Work out the finished part from the listing and answer in its coordinate system (mm). A direction names the side the tool comes from. Give positions to 0.01 mm unless a question says otherwise; leave off trailing zeros. Loops run counter-clockwise (first coordinate to the right, second up) from the corner with the lowest first, then second, coordinate; pieces in that order, holes last. Notation, with made-up numbers: M 78,-34 L 100,-34 A26 ccw 100,-10 Z; hole C -29,-37 d5. An arc over 180 degrees is marked long. Answer in a Markdown table with one row per item. Add a question column.
from build123d import *

# Parameters (mm, degrees)
SKETCH2_W           = 130
SKETCH2_H           = 40
BOSS_EXTRUDE1_DEPTH = 75
SKETCH6_W           = 29.16
SKETCH6_H           = 49.32
BOSS_EXTRUDE2_DEPTH = 16.07
SKETCH7_W           = 15.96
SKETCH7_H           = 42.65
CUT_EXTRUDE1_DEPTH  = 8.48
SKETCH8_W           = 7
SKETCH8_H           = 42.65
CUT_EXTRUDE2_DEPTH  = 1.145
SKETCH9_W           = 7
SKETCH9_H           = 42.65
CUT_EXTRUDE3_DEPTH  = 1.145
SKETCH11_W          = 35.86
SKETCH11_H          = 21.1
CUT_EXTRUDE4_DEPTH  = 8.2
SKETCH13_W          = 3.9
SKETCH13_H          = 21.1
CUT_EXTRUDE5_DEPTH  = 1.145
SKETCH14_W          = 3.9
SKETCH14_H          = 21.1
CUT_EXTRUDE6_DEPTH  = 1.145
SKETCH15_W          = 35.86
SKETCH15_H          = 21.1
CUT_EXTRUDE7_DEPTH  = 8.2
SKETCH16_W          = 3.9
SKETCH16_H          = 21.1
CUT_EXTRUDE8_DEPTH  = 1.145
SKETCH17_W          = 3.9
SKETCH17_H          = 21.1
CUT_EXTRUDE9_DEPTH  = 1.145
SKETCH20_W          = 29.16
SKETCH20_H          = 16.07
BOSS_EXTRUDE3_DEPTH = 25.68
SKETCH21_W          = 40
SKETCH21_H          = 25
CUT_EXTRUDE10_DEPTH = 40
SKETCH22_W          = 50
SKETCH22_H          = 25
CUT_EXTRUDE11_DEPTH = 40
BOSS_EXTRUDE4_DEPTH = 8
BOSS_EXTRUDE5_DEPTH = 8


with BuildPart() as part:
    # Sketch2 → Boss-Extrude1 (new body)
    with BuildSketch(Plane(origin=(0, 0, 0), x_dir=(1, 0, 0), z_dir=(0, 1, 0))):
        Rectangle(SKETCH2_W, SKETCH2_H)
    extrude(amount=BOSS_EXTRUDE1_DEPTH)

    # Sketch6 → Boss-Extrude2 (add)
    with BuildSketch(Plane.XY.offset(20)):
        with Locations((0, 50.34)):
            Rectangle(SKETCH6_W, SKETCH6_H)
    extrude(amount=BOSS_EXTRUDE2_DEPTH)

    # Sketch7 → Cut-Extrude1 (cut)
    with BuildSketch(Plane.XY.offset(36.07)):
        with Locations((0, 53.675)):
            Rectangle(SKETCH7_W, SKETCH7_H)
    extrude(amount=-CUT_EXTRUDE1_DEPTH, mode=Mode.SUBTRACT)

    # Sketch8 → Cut-Extrude2 (cut)
    with BuildSketch(Plane(origin=(-7.98, 0, 0), x_dir=(0, 0, -1), z_dir=(1, 0, 0))):
        with Locations((-31.09, 53.675)):
            Rectangle(SKETCH8_W, SKETCH8_H)
    extrude(amount=-CUT_EXTRUDE2_DEPTH, mode=Mode.SUBTRACT)

    # Sketch9 → Cut-Extrude3 (cut)
    with BuildSketch(Plane.ZY.offset(-7.98)):
        with Locations((31.09, 53.675)):
            Rectangle(SKETCH9_W, SKETCH9_H)
    extrude(amount=-CUT_EXTRUDE3_DEPTH, mode=Mode.SUBTRACT)

    # Sketch11 → Cut-Extrude4 (cut)
    with BuildSketch(Plane.XY.offset(20)):
        with Locations((42.64, 64.45)):
            Rectangle(SKETCH11_W, SKETCH11_H)
    extrude(amount=-CUT_EXTRUDE4_DEPTH, mode=Mode.SUBTRACT)

    # Sketch13 → Cut-Extrude5 (cut)
    with BuildSketch(Plane(origin=(24.71, 0, 0), x_dir=(0, 0, -1), z_dir=(1, 0, 0))):
        with Locations((-13.75, 64.45)):
            Rectangle(SKETCH13_W, SKETCH13_H)
    extrude(amount=-CUT_EXTRUDE5_DEPTH, mode=Mode.SUBTRACT)

    # Sketch14 → Cut-Extrude6 (cut)
    with BuildSketch(Plane.ZY.offset(-60.57)):
        with Locations((13.75, 64.45)):
            Rectangle(SKETCH14_W, SKETCH14_H)
    extrude(amount=-CUT_EXTRUDE6_DEPTH, mode=Mode.SUBTRACT)

    # Sketch15 → Cut-Extrude7 (cut)
    with BuildSketch(Plane.XY.offset(20)):
        with Locations((-42.64, 64.45)):
            Rectangle(SKETCH15_W, SKETCH15_H)
    extrude(amount=-CUT_EXTRUDE7_DEPTH, mode=Mode.SUBTRACT)

    # Sketch16 → Cut-Extrude8 (cut)
    with BuildSketch(Plane(origin=(-60.57, 0, 0), x_dir=(0, 0, -1), z_dir=(1, 0, 0))):
        with Locations((-13.75, 64.45)):
            Rectangle(SKETCH16_W, SKETCH16_H)
    extrude(amount=-CUT_EXTRUDE8_DEPTH, mode=Mode.SUBTRACT)

    # Sketch17 → Cut-Extrude9 (cut)
    with BuildSketch(Plane.ZY.offset(24.71)):
        with Locations((13.75, 64.45)):
            Rectangle(SKETCH17_W, SKETCH17_H)
    extrude(amount=-CUT_EXTRUDE9_DEPTH, mode=Mode.SUBTRACT)

    # Sketch20 → Boss-Extrude3 (add)
    with BuildSketch(Plane(origin=(0, 25.68, 0), x_dir=(-1, 0, 0), z_dir=(0, -1, 0))):
        with Locations((0, -28.035)):
            Rectangle(SKETCH20_W, SKETCH20_H)
    extrude(amount=BOSS_EXTRUDE3_DEPTH)

    # Sketch21 → Cut-Extrude10 (cut)
    with BuildSketch(Plane(origin=(0, 75, 0), x_dir=(1, 0, 0), z_dir=(0, 1, 0))):
        with Locations((45, 7.5)):
            Rectangle(SKETCH21_W, SKETCH21_H)
        with Locations((-45, 7.5)):
            Rectangle(SKETCH21_W, SKETCH21_H)
    extrude(amount=-CUT_EXTRUDE10_DEPTH, mode=Mode.SUBTRACT)

    # Sketch22 → Cut-Extrude11 (cut)
    with BuildSketch(Plane(origin=(0, 75, 0), x_dir=(1, 0, 0), z_dir=(0, 1, 0))):
        with Locations((0, 7.5)):
            Rectangle(SKETCH22_W, SKETCH22_H)
    extrude(amount=-CUT_EXTRUDE11_DEPTH, mode=Mode.SUBTRACT)

    # Sketch23 → Boss-Extrude4 (add)
    with BuildSketch(Plane(origin=(0, 53.9, 0), x_dir=(1, 0, 0), z_dir=(0, 1, 0))):
        Polygon((-60.57, -20), (-60.57, -15.7), (-61.715, -15.7), (-61.715, -11.8), (-23.565, -11.8), (-23.565, -15.7), (-24.71, -15.7), (-24.71, -20), align=None)
    extrude(amount=BOSS_EXTRUDE4_DEPTH)

    # Sketch24 → Boss-Extrude5 (add)
    with BuildSketch(Plane(origin=(0, 53.9, 0), x_dir=(1, 0, 0), z_dir=(0, 1, 0))):
        Polygon((24.71, -20), (24.71, -15.7), (23.565, -15.7), (23.565, -11.8), (61.715, -11.8), (61.715, -15.7), (60.57, -15.7), (60.57, -20), align=None)
    extrude(amount=BOSS_EXTRUDE5_DEPTH)


solid = part.part
(1) Section B-B, the plane y = 48.5 is taken. Determine the outline of the cut face in (x, z) (3 decimals).
(2) Section C-C, the plane z = 23.5 is taken. Determine the outline of the cut face in (x, y), and give its area (3 significant figures).
(3) Section A-A, the plane x = 52.5 is taken. Determine the outline of the cut face in (y, z), and give its area (3 significant figures).
(4) Each of these flat-tipped pins is pushed along its axis until it touches: P1, Ø0.9, axis at x = -61.5, y = 67, coming from the -Z side; P2, Ø1.2, axis at y = 45.5, z = 35.5, coming from the -X side; P3, Ø20, axis at x = -29.5, z = -9.5, coming from the +Y side. Where does it stop, or does it pass through?
(5) The mould has two halves that part along X. Classify faces 6 (the face through (-65, 29, 5)), 7 (the face through (1, 0, 1)), 8 (the face through (42, 68, 11.8)): pulls with the +X half, pulls with the -X half, needs draft (parallel to the pull), parting line crosses it, or undercut.
(6) Consider line 1 along X through (y, z) = (44, 28) (3 decimals); line 2 along X through (y, z) = (17.5, 23); line 3 along Y through (x, z) = (-34.5, 0). Determine where each line is inside the solid, lowest interval first. Write a range as from..to.
(7) Section D-D, the plane y = 6.5 is taken. Determine the outline of the cut face in (x, z), and give its area (3 significant figures).
(8) Which of the six approach directions +Z, -Z, +X, -X, +Y, -Y give full straight-line access (tool end or side, diameter ignored) to faces 1 (the face through (14.58, 38, 28)), 2 (the face through (-60.57, 68, 18)), 3 (the face through (-61.715, 69, 14)), 4 (the face through (-14.58, 38, 28)), 5 (the face through (-1, 35, -8))?
Numbers:
| question | item | result |
|---|---|---|
| 1 | outline | M -65,5 L 65,5 L 65,20 L 14.58,20 L 14.58,36.07 L 7.98,36.07 L 7.98,34.59 L 9.125,34.59 L 9.125,27.59 L -9.125,27.59 L -9.125,34.59 L -7.98,34.59 L -7.98,36.07 L -14.58,36.07 L -14.58,20 L -65,20 Z |
| 2 | outline | M -14.58,0 L 14.58,0 L 14.58,75 L -14.58,75 Z |
| 2 | area | 2,190 mm² |
| 3 | outline | M 0,-20 L 35,-20 L 35,5 L 75,5 L 75,11.8 L 61.9,11.8 L 61.9,20 L 0,20 Z |
| 3 | area | 1,890 mm² |
| 4 | P1 | stops at z = 5 |
| 4 | P2 | stops at x = -14.58 |
| 4 | P3 | stops at y = 35 |
| 5 | face 6 | pulls with the -X half |
| 5 | face 7 | needs draft |
| 5 | face 8 | undercut |
| 6 | line 1 | x = -14.58..-9.125, 9.125..14.58 |
| 6 | line 2 | x = -14.58..14.58 |
| 6 | line 3 | y = 0..35 |
| 7 | outline | M -65,-20 L 65,-20 L 65,20 L 14.58,20 L 14.58,36.07 L -14.58,36.07 L -14.58,20 L -65,20 Z |
| 7 | area | 5,670 mm² |
| 8 | face 1 | +Z, +X, +Y, -Y |
| 8 | face 2 | +Z, +Y |
| 8 | face 3 | +Y |
| 8 | face 4 | +Z, -X, +Y, -Y |
| 8 | face 5 | -Z, +X, -X, +Y |
